```python
from build123d import *

# Parameters (mm, degrees)
F1_DEPTH = 25.4
F2_W     = 3.5091163591
F2_H     = 4.6407710761
F3_DEPTH = 0.0254


with BuildPart() as f1:
    # F0 (on Top) → F1 (new body)
    with BuildSketch(Plane.XY):
        Polygon((-15.5386179686, 51.1961877346), (-48.8319955766, 60.7384853065), (-49.6143862535, 57.6021264383), (-76.441437006, -49.9391071498), (-86.0654970387, -83.5177565662), (-76.441437006, -85.4337778982), (-55.8721683804, -89.5288435292), (-38.5488659292, -29.0872941455), (-22.0129852453, 28.6069158224), align=None)
        Polygon((-49.6143862535, 57.6021264383), (-48.8319955766, 60.7384853065), (-72.3904520273, 43.7064096332), (-94.5257858226, -33.524469091), (-97.1982382925, -44.2374929704), (-93.384412075, -57.6940258869), (-86.0654970387, -83.5177565662), (-76.441437006, -49.9391071498), align=None)
        Polygon((-99.0511800836, -53.5447082589), (-86.0654970387, -83.5177565662), (-93.384412075, -57.6940258869), (-97.1982382925, -44.2374929704), align=None)
    extrude(amount=F1_DEPTH)

    # F2 (on face) → F3 (join)
    with BuildSketch(Plane(origin=(-78.4711106248, 22.4907997378, 0), x_dir=(-0.2755193001, -0.96129554, 0), z_dir=(-0.96129554, 0.2755193001, 0))):
        with Locations((-12.2740664519, 15.7686183229)):
            Rectangle(F2_W, F2_H)
    extrude(amount=F3_DEPTH)


solid = f1.part
```
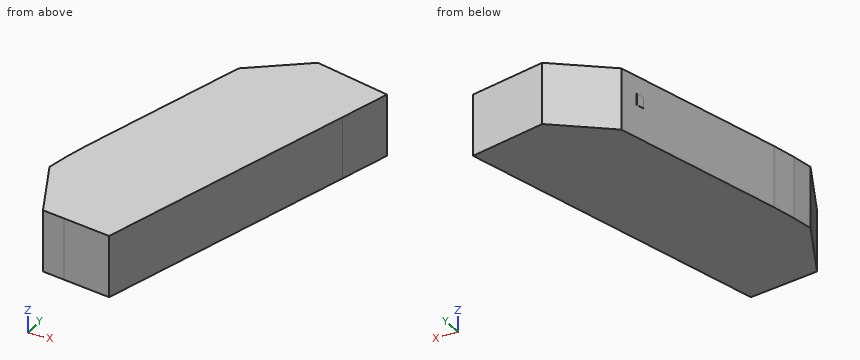
The model under review builds one solid part; all positions refer to its coordinate system, in mm. Round coordinates to 2 decimals unless told otherwise and drop trailing zeros. Loops run counter-clockwise (first coordinate to the right, second up) from the corner with the lowest first, then second, coordinate; pieces in that order, holes last. Notation, with made-up numbers: (-31.5, -30.5) -> (-23.5, -30.5) arc R25 ccw to (-23.5, -4.5) -> close; hole circle Ø3 at (57, 0.5). An arc over 180 degrees is marked (long way). Answer as a JSON object with one key per item and string values. Group by question number.
1) We need section C-C on x = -68. Write out the cut boundary in (y, z).
2) We need section D-D on y = 40.5. Write out the cut boundary in (x, z), then the cut area to 3 significant figures.
3) For pin 1 Ø1.5 at (y, z) = (-39, 9.5) entering from +X (3 decimals); pin 2 Ø10 at (x, z) = (-28.5, 12.5) entering from +Y; pin 3 Ø1 at (y, z) = (-59.5, 5.5) entering from -X, all flat-tipped, find the tip position at first contact; note any pin that passes through.
4) We need section A-A on z = 6.75. Write out the cut boundary in (x, y), then the cut area to 3 significant figures.
5) For line 1 (X direction, y = -68.5, z = 11); line 2 (X direction, y = 32, z = 13.75); line 3 (Y direction, x = -66, z = 2.5), list the stretches that pass through material, from the lowest coordinate up. Write a range as [from, to].
Result set:
{
 "1": {"outline": "(-87.11, 0) -> (46.88, 0) -> (46.88, 25.4) -> (-87.11, 25.4) -> close"},
 "2": {"outline": "(-73.31, 0) -> (-18.6, 0) -> (-18.6, 25.4) -> (-73.31, 25.4) -> close", "area": "1,390 mm²"},
 "3": {"pin 1": "x = -41.175", "pin 2": "y = 56.34", "pin 3": "x = -96.69"},
 "4": {"outline": "(-99.05, -53.54) -> (-86.07, -83.52) -> (-55.87, -89.53) -> (-15.54, 51.2) -> (-48.83, 60.74) -> (-72.39, 43.71) -> (-94.53, -33.52) -> (-97.2, -44.24) -> close", "area": "7,290 mm²"},
 "5": {"line 1": "[-92.57, -49.85]", "line 2": "[-75.75, -21.04]", "line 3": "[-87.51, 48.33]"}
}
